Source: CAD feature listing. Evaluate the final solid. Frame: model axes, mm. Face numbers are marked on the shaded views. Round coordinates to 2 decimals unless told otherwise and drop trailing zeros. Order: outer loops, then holes, each group sorted by start corner. A loop starts at its lowest first (then second) coordinate and runs counter-clockwise, first axis right, second up. Notation, with made-up numbers: (82, 49) -> (95, 49) arc R24 cw to (95, 82) -> close; hole circle Ø8 at (50.5, 14.25). An arc over 180 degrees is marked (long way). Answer as CSV lines item,"result".
from build123d import *

# Parameters (mm, degrees)
M6_CLEARANCE_HOLE1_D = 6.74624
M6_CLEARANCE_HOLE2_D = 6.74624
CHAMFER1_SIZE        = 0.18288
CHAMFER2_SIZE        = 0.889


with BuildPart() as part:
    # Sketch1 → Revolve1 (revolve)
    with BuildSketch(Plane(origin=(0, 0, 0), x_dir=(-1, 0, 0), z_dir=(0, 0, -1)), mode=Mode.PRIVATE) as revolve1_sk:
        Polygon((-5.08, 20.955), (-5.08, 0), (6.35, 0), (6.35, 34.671), (2.54, 34.671), (2.54, 33.0835), (-2.54, 33.0835), (-2.54, 34.671), (-6.35, 34.671), (-6.35, 24.13), (-4.559394506, 24.13), (-5.715, 20.955), align=None)
    revolve(revolve1_sk.sketch.rotate(Axis((6.35, 0, 0), (-1, 0, 0)), 270), axis=Axis((6.35, 0, 0), (-1, 0, 0)))

    # M6 Clearance Hole1 (through all)
    with Locations(Plane(origin=(6.35, 0, 0), x_dir=(0, 0, -1), z_dir=(1, 0, 0))):
        with Locations((0, 29.36875), (25.434083577, 14.684375), (0, -29.36875), (-25.434083577, 14.684375)):
            Hole(M6_CLEARANCE_HOLE1_D / 2)

    # M6 Clearance Hole2 (through all)
    with Locations(Plane.ZY.offset(6.35)):
        with Locations((25.434083577, -14.684375), (-25.434083577, -14.684375)):
            Hole(M6_CLEARANCE_HOLE2_D / 2)

    # Chamfer1
    chamfer1_edges = [part.edges().sort_by_distance(p)[0] for p in [
        (6.35, 14.684375, 22.060963577),
        (-6.35, 14.684375, 22.060963577),
        (6.35, -29.36875, -3.37312),
        (-6.35, -29.36875, -3.37312),
        (6.35, 14.684375, -28.807203577),
        (-6.35, 14.684375, -28.807203577),
        (6.35, 29.36875, -3.37312),
        (-6.35, 29.36875, -3.37312),
        (-6.35, -14.684375, -22.060963577),
        (6.35, -14.684375, -22.060963577),
        (-6.35, -14.684375, 28.807203577),
        (6.35, -14.684375, 28.807203577),
    ]]
    chamfer(chamfer1_edges, length=CHAMFER1_SIZE)

    # Chamfer2
    chamfer2_edges = [part.edges().sort_by_distance(p)[0] for p in [
        (6.35, 0, -34.671),
        (-6.35, 0, -34.671),
    ]]
    chamfer(chamfer2_edges, length=CHAMFER2_SIZE)


solid = part.part
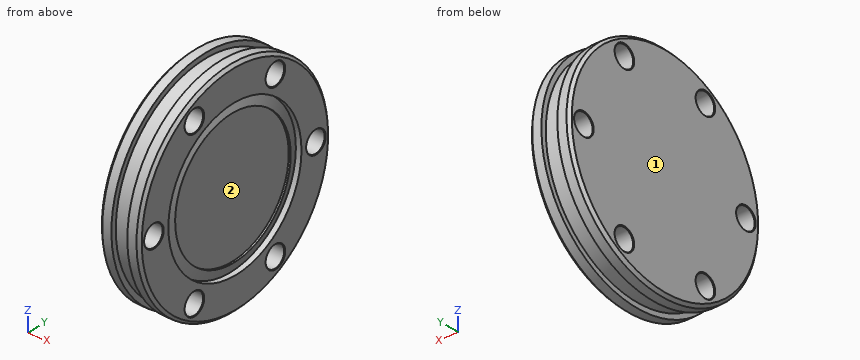
1. Mould query, pull axis Y, two halves, no side actions, for the marked faces 1 and 2. Classes: released by +Y, released by -Y, zero draft, split by the parting line, or undercut.
Results below:
face 1,"zero draft"
face 2,"undercut"
2. Section query C-C on z = 0. Give the number of separate pieces and of enclosed holes in the cut face, and give its area (3 significant figures).
Results below:
separate pieces,"3"
enclosed holes,"0"
area,"631 mm2"
3. Line query: L1, parallel to Y at x = -0.25, z = 0; L2, parallel to Y at x = 4.5, z = -24; L3, parallel to Z at x = 2.5, y = 16.5. Output: solid intervals per line, ascending. Write a range as [from, to].
Results below:
L1,"[-33.08, -32.74], [-26, 26], [32.74, 33.08]"
L2,"[-25.02, -17.74], [-11.63, 11.63], [17.74, 25.02]"
L3,"[-28.68, -28.28], [-22.59, 22.59], [28.28, 28.68]"
4. Pin query (flat end, axial travel): pin 1 (3 mm diameter, centred on y = -11, z = -7.5, fed in from +X); pin 2 (3 mm diameter, centred on x = 2, z = 23, fed in from -Y); pin 3 (2 mm diameter, centred on x = 3, y = 1.5, fed in from -Z). Return the tip coordinate at first contact, or that it passes through.
Results below:
pin 1,"x = 5.08"
pin 2,"y = -27.12"
pin 3,"z = -34.67"
5. Section query B-B on x = -4.25. Return loops of the section in (y, z), and give its area (3 significant figures).
Results below:
outline,"circle Ø69.34 at (0, 0); hole circle Ø6.75 at (-29.37, 0); hole circle Ø6.75 at (-14.68, -25.43); hole circle Ø6.75 at (-14.68, 25.43); hole circle Ø6.75 at (14.68, -25.43); hole circle Ø6.75 at (14.68, 25.43); hole circle Ø6.75 at (29.37, 0)"
area,"3,560 mm2"
